Solid Edge part; units mm, degrees
sketch "Sketch1" plane through (0, 0, 0) normal (0, -1, 0) x (1, 0, 0)
  line L0 (100.1511, 54) -> (100.1511, 0)
  line L1 (100.1511, 0) -> (0, 0)
  line L2 (0, 0) -> (0, 54)
  line L3 (0, 54) -> (100.1511, 54)
extrude "Protrusion1" add sketch "Sketch1" along normal blind 3.7656
sketch "Sketch2" plane through (50.0756, -3.7656, 27) normal (0, -1, 0) x (1, 0, 0)
  line L0 (40.4, -15.04) -> (-43.76, -15.04)
  line L1 (-43.76, -15.04) -> (-43.76, 18.24)
  line L2 (-43.76, 18.24) -> (40.4, 18.24)
  line L3 (40.4, 18.24) -> (40.4, -15.04)
extrude "Cutout1" cut sketch "Sketch2" against normal blind 1.7665
Can you work these out from the model? Positions are in its coordinate system, mm. A direction names the side the tool comes from. Round coordinates to 2 decimals unless told otherwise and drop trailing zeros. Write each loop counter-clockwise with the first axis right and the second up, starting at its lowest first coordinate (ties: lowest second). Pieces come first, ordered by that corner, then holes. Notation, with made-up numbers: (-1.75, 54) - (51.25, 54) arc R14 ccw to (51.25, 62) - close; hole circle Ø1 at (-32, 20). An arc over 180 degrees is marked (long way). Write each question's results on one line, items separated by ' | '. Start each with the question number.
1) Please list where these lines run through material, in increasing order: line 1 (Z direction, x = 32.5, y = -3.2); line 2 (X direction, y = -3.3, z = 38); line 3 (Y direction, x = 66, z = 34).
2) Suppose I cut it at A-A (z = 24). List the corners of the cut face in (x, y) for me, and give its area (3 significant figures).
3) We'd pull the mould along Z, two halves only. Please class faces 1 (the flat face through (51, -2, 0)), 2 (the flat face through (48, -3, 45.24)), 3 (the flat face through (100.151, -2, 27)), 4 (the flat face through (49, -3, 11.96)): released by +Z, released by -Z, zero draft, split by the parting line, or undercut.
4) Suppose I cut it at B-B (x = 81.5). List the corners of the cut face in (y, z) for me, and give its area (3 significant figures).
5) For pin 1 Ø2 at (x, z) = (22, 47) entering from +Y; pin 2 Ø10 at (x, z) = (69.5, 27) entering from -Y, each with a flat end and sliding along its axis, tell me the tip position at first contact or that it passes through.
6) Which directions (+Z, -Z, +X, -X, +Y, -Y) give clear straight access to the entire face, cutting with the end or side of a thin tool? Please do faces 5 (the flat face through (49, -2, 54)), 6 (the flat face through (90.476, -3, 29)).
Here are the results:
1) line 1: z = 0 to 11.96, 45.24 to 54 | line 2: x = 0 to 6.32, 90.48 to 100.15 | line 3: y = -2 to 0
2) outline: (0, -3.77) - (6.32, -3.77) - (6.32, -2) - (90.48, -2) - (90.48, -3.77) - (100.15, -3.77) - (100.15, 0) - (0, 0) - close | area: 228 mm2
3) face 1: released by -Z | face 2: undercut | face 3: zero draft | face 4: undercut
4) outline: (-3.77, 0) - (0, 0) - (0, 54) - (-3.77, 54) - (-3.77, 45.24) - (-2, 45.24) - (-2, 11.96) - (-3.77, 11.96) - close | area: 145 mm2
5) pin 1: stops at y = 0 | pin 2: stops at y = -2
6) face 5: +Z, +X, -X, +Y, -Y | face 6: -Y
